Autodesk Inventor part; units mm, degrees
ref_plane "YZ Plane" through (0, 0, 0) normal (1, 0, 0) x (0, 1, 0)
ref_plane "XZ Plane" through (0, 0, 0) normal (0, 1, 0) x (-1, 0, 0)
ref_plane "XY Plane" through (0, 0, 0) normal (0, 0, 1) x (1, 0, 0)
sketch "Sketch1" plane through (0, 0, 0) normal (0, 0, 1) x (1, 0, 0)
  line L0 (-12.7, -25.4) -> (12.7, -25.4)
  line L1 (12.7, -25.4) -> (12.7, 25.4)
  line L2 (12.7, 25.4) -> (-12.7, 25.4)
  line L3 (-12.7, 25.4) -> (-12.7, -25.4)
  line L4 (-12.7, -25.4) -> (12.7, 25.4) construction
  line L5 (12.7, -25.4) -> (-12.7, 25.4) construction
  line L6 (-10.16, -22.86) -> (10.16, -22.86)
  line L7 (10.16, -22.86) -> (10.16, 22.86)
  line L8 (10.16, 22.86) -> (-10.16, 22.86)
  line L9 (-10.16, 22.86) -> (-10.16, -22.86)
  line L10 (-10.16, -22.86) -> (10.16, 22.86) construction
  line L11 (10.16, -22.86) -> (-10.16, 22.86) construction
  point P0 (0, 0)
  dimension "d0" = 25.4
  dimension "d1" = 50.8
  dimension "d2" = 20.32
  dimension "d3" = 45.72
extrude "Extrusion1" add sketch "Sketch1" along normal mid plane 177.8
sketch "Sketch2" plane through (-12.7, 25.4, 88.9) normal (0, 1, 0) x (1, 0, 0)
  line L0 (25.4, 177.8) -> (25.4, 0)
  line L1 (25.4, 0) -> (0, 0)
  point P0 (12.7, 88.9)
  point P1 (12.7, 12.7)
  dimension "d6" = 12.7
  dimension "d7" = 12.7
hole "Hole1" at (0, 25.4, 76.2) direction (0, -1, 0) diameter 4.1402 end through all
pattern_linear "Rectangular Pattern1" count 7 spacing 25.4 along (0, 0, -1) of "Hole1"
sketch "Sketch3" plane through (12.7, -25.4, 88.9) normal (1, 0, 0) x (0, 0, -1)
  line L0 (0, 0) -> (0, 50.8)
  line L1 (177.8, 0) -> (0, 0)
  point P0 (88.9, 25.4)
  point P1 (17.625, 25.4)
  dimension "d18" = 17.625
  dimension "d19" = 25.4
hole "Hole2" at (12.7, 0, 71.275) direction (-1, 0, 0) diameter 28.5496 end through all
sketch "Sketch4" plane through (12.7, -25.4, 88.9) normal (1, 0, 0) x (0, 0, -1)
  point P0 (88.9, 25.4)
  point P1 (144.3097, 40.5612)
  point P2 (169.7097, 40.5612)
  point P3 (169.7097, 15.1612)
  point P4 (144.3097, 15.1612)
  dimension "d27" = 25.4
  dimension "d28" = 25.4
hole "Hole3" at (12.7, 15.1612, -55.4097) at (12.7, 15.1612, -80.8097) at (12.7, -10.2388, -80.8097) at (12.7, -10.2388, -55.4097) direction (-1, 0, 0) diameter 4.1402 end through all
properties part number "Horizontal_intake_hanger"
Check sheet for the modelled part. Datum: model origin and axes. Units: mm. A direction names the side the tool comes from. Round coordinates to 2 decimals unless told otherwise and drop trailing zeros. Order: outer loops, then holes, each group sorted by start corner. A loop starts at its lowest first (then second) coordinate and runs counter-clockwise, first axis right, second up.
(1) Access from +Z, -Z, +X, -X, +Y, -Y to the whole of each face (thin tool, end or side, straight path). Record for faces 5 (the flat face through (2, -22.86, -1)), 6 (the cylindrical face through (11.41, 15.07, -78.74)).
(2) Cross-section at C-C, the plane z = -10. Enter the section's corners in (x, y).
(3) Cross-section at A-A, the plane y = 0. Enter the section's corners in (x, z).
(4) Cross-section at D-D, the plane z = 76.2. Enter the section's corners in (x, y), and give its area (3 significant figures).
(5) Draft check along Y on faces 1 (the cylindrical face through (-0.09, -24.15, -52.87)), 2 (the cylindrical face through (-11.45, -10.33, -78.74)), 3 (the flat face through (-3, 25.4, -1)), 4 (the cylindrical face through (11.412, 15.954, -57.322)). Enter one of: pulls with the +Y half, pulls with the -Y half, needs draft (parallel to the pull), parting line crosses it, or undercut.
(6) Cross-section at B-B, the plane x = 4.75. Enter the section's corners in (y, z), and give its area (3 significant figures).
(7) Scan lines: probe 1 along X at (y, z) = (23.8, 0); probe 2 along X at (y, z) = (12, -57); probe 3 along Y at (x, z) = (-2.5, -45). Record each from-to range of solid material in increasing order.
Check sheet entries:
1. face 5: +Z, -Z
1. face 6: +X, -X
2. outline: (-12.7, -25.4) - (12.7, -25.4) - (12.7, 25.4) - (-12.7, 25.4) - close; hole (-10.16, -22.86) - (10.16, -22.86) - (10.16, 22.86) - (-10.16, 22.86) - close
3. outline: (-12.7, -88.9) - (-10.16, -88.9) - (-10.16, 57) - (-12.7, 57) - close; (-12.7, 85.55) - (-10.16, 85.55) - (-10.16, 88.9) - (-12.7, 88.9) - close; (10.16, -88.9) - (12.7, -88.9) - (12.7, 57) - (10.16, 57) - close; (10.16, 85.55) - (12.7, 85.55) - (12.7, 88.9) - (10.16, 88.9) - close
4. outline: (-12.7, -25.4) - (-2.07, -25.4) - (-2.07, -22.86) - (-10.16, -22.86) - (-10.16, -13.4) - (-12.7, -13.4) - close; (-12.7, 13.4) - (-10.16, 13.4) - (-10.16, 22.86) - (-2.07, 22.86) - (-2.07, 25.4) - (-12.7, 25.4) - close; (2.07, -25.4) - (12.7, -25.4) - (12.7, -13.4) - (10.16, -13.4) - (10.16, -22.86) - (2.07, -22.86) - close; (2.07, 22.86) - (10.16, 22.86) - (10.16, 13.4) - (12.7, 13.4) - (12.7, 25.4) - (2.07, 25.4) - close
4. area: 204 mm2
5. face 1: needs draft
5. face 2: undercut
5. face 3: pulls with the +Y half
5. face 4: undercut
6. outline: (-25.4, -88.9) - (-22.86, -88.9) - (-22.86, 88.9) - (-25.4, 88.9) - close; (22.86, -88.9) - (25.4, -88.9) - (25.4, 88.9) - (22.86, 88.9) - close
6. area: 903 mm2
7. probe 1: x = -12.7 to -2.07, 2.07 to 12.7
7. probe 2: x = -12.7 to -10.16, 10.16 to 12.7
7. probe 3: y = -25.4 to -22.86, 22.86 to 25.4
